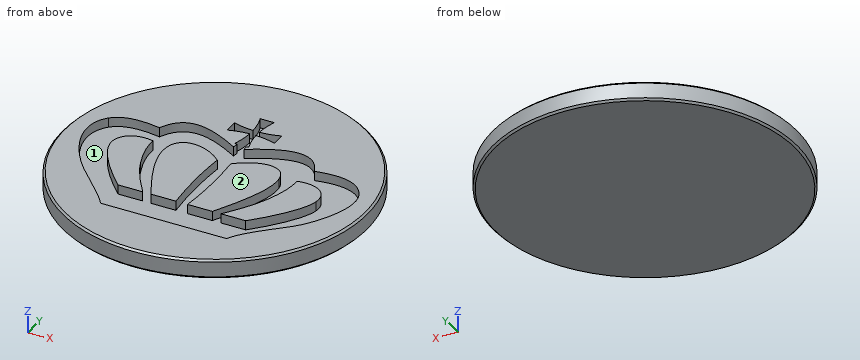
from build123d import *

# Parameters (mm, degrees)
POCKET_DEPTH = 1.25


with BuildPart() as part:
    # Sketch (on DatumPlane) → Revolution (revolve)
    with BuildSketch(Plane.YZ):
        Polygon((0, 0), (0, -2.5), (19.75, -2.5), (20, -2.25), (20, -0.25), (19.75, 0), align=None)
    revolve(axis=Axis((0, 0, 0), (0, 0, 1)))

    # Sketch005 → Pocket (cut)
    with BuildSketch(Plane.XY):
        with BuildLine():
            add(Edge.make_bspline(
                [(17.199673, 3.39502), (15.904895, 5.827494), (13.139208, 6.003619), (10.22119, 5.380033)],
                knots=[0, 0, 0, 0, 1, 1, 1, 1], degree=3))
            add(Edge.make_bspline(
                [(10.22119, 5.380033), (8.593193, 9.516663), (4.81358, 8.293289), (0.719788, 5.827494)],
                knots=[0, 0, 0, 0, 1, 1, 1, 1], degree=3))
            add(Edge.make_bspline(
                [(0.719788, 5.827494), (0.649422, 6.478351)],
                knots=[0, 0, 41.237809, 41.237809], degree=1))
            add(Edge.make_bspline(
                [(0.649422, 6.478351), (0.817118, 6.478351), (0.936272, 6.478351), (0.959337, 6.478351)],
                knots=[0, 0, 0, 0, 1, 1, 1, 1], degree=3))
            add(Edge.make_bspline(
                [(0.959337, 6.478351), (0.65764, 7.35953), (0.487238, 8.273468), (0.447992, 9.191671)],
                knots=[0, 0, 0, 0, 1, 1, 1, 1], degree=3))
            add(Edge.make_bspline(
                [(0.447992, 9.191671), (1.366194, 9.152423), (2.280132, 8.982021), (3.16131, 8.680326)],
                knots=[0, 0, 0, 0, 1, 1, 1, 1], degree=3))
            add(Edge.make_bspline(
                [(3.16131, 8.680326), (3.16131, 9.295984), (3.16131, 9.911639), (3.16131, 10.527295)],
                knots=[0, 0, 0, 0, 1, 1, 1, 1], degree=3))
            add(Edge.make_bspline(
                [(3.16131, 10.527295), (2.280132, 10.225599), (1.366194, 10.055198), (0.447992, 10.01595)],
                knots=[0, 0, 0, 0, 1, 1, 1, 1], degree=3))
            add(Edge.make_bspline(
                [(0.447992, 10.01595), (0.487238, 10.934154), (0.65764, 11.848094), (0.959337, 12.729271)],
                knots=[0, 0, 0, 0, 1, 1, 1, 1], degree=3))
            add(Edge.make_bspline(
                [(0.959337, 12.729271), (0.343681, 12.729271), (-0.271977, 12.729271), (-0.887634, 12.729271)],
                knots=[0, 0, 0, 0, 1, 1, 1, 1], degree=3))
            add(Edge.make_bspline(
                [(-0.887634, 12.729271), (-0.585937, 11.848092), (-0.415537, 10.934152), (-0.376289, 10.01595)],
                knots=[0, 0, 0, 0, 1, 1, 1, 1], degree=3))
            add(Edge.make_bspline(
                [(-0.376289, 10.01595), (-1.294491, 10.055198), (-2.20843, 10.2256), (-3.089607, 10.527295)],
                knots=[0, 0, 0, 0, 1, 1, 1, 1], degree=3))
            add(Edge.make_bspline(
                [(-3.089607, 10.527295), (-3.089607, 9.911639), (-3.089607, 9.295983), (-3.089607, 8.680326)],
                knots=[0, 0, 0, 0, 1, 1, 1, 1], degree=3))
            add(Edge.make_bspline(
                [(-3.089607, 8.680326), (-2.20843, 8.982023), (-1.294491, 9.152423), (-0.376289, 9.191671)],
                knots=[0, 0, 0, 0, 1, 1, 1, 1], degree=3))
            add(Edge.make_bspline(
                [(-0.376289, 9.191671), (-0.415537, 8.273468), (-0.585937, 7.359528), (-0.887634, 6.478351)],
                knots=[0, 0, 0, 0, 1, 1, 1, 1], degree=3))
            add(Edge.make_bspline(
                [(-0.887634, 6.478351), (-0.857358, 6.478351), (-0.732021, 6.478351), (-0.559748, 6.478351)],
                knots=[0, 0, 0, 0, 1, 1, 1, 1], degree=3))
            add(Edge.make_bspline(
                [(-0.559748, 6.478351), (-0.641636, 5.73229)],
                knots=[0, 0, 47.278241, 47.278241], degree=1))
            add(Edge.make_bspline(
                [(-0.641636, 5.73229), (-4.754593, 8.196928), (-8.497006, 9.617448), (-10.238244, 5.399072)],
                knots=[0, 0, 0, 0, 1, 1, 1, 1], degree=3))
            add(Edge.make_bspline(
                [(-10.238244, 5.399072), (-12.781371, 5.921869), (-15.207916, 5.846532), (-16.502695, 4.485108)],
                knots=[0, 0, 0, 0, 1, 1, 1, 1], degree=3))
            add(Edge.make_bspline(
                [(-16.502695, 4.485108), (-19.031136, 1.826532), (-16.97872, -3.140769), (-13.656084, -6.796618)],
                knots=[0, 0, 0, 0, 1, 1, 1, 1], degree=3))
            add(Edge.make_bspline(
                [(-13.656084, -6.796618), (-11.875374, -8.755908), (-9.359237, -11.018558), (-8.286551, -12.670729)],
                knots=[0, 0, 0, 0, 1, 1, 1, 1], degree=3))
            add(Edge.make_bspline(
                [(-8.286551, -12.670729), (8.364704, -12.670729)],
                knots=[0, 0, 1048.89791, 1048.89791], degree=1))
            add(Edge.make_bspline(
                [(8.364704, -12.670729), (9.202504, -10.757117), (12.053892, -8.352741), (13.859035, -6.607594)],
                knots=[0, 0, 0, 0, 1, 1, 1, 1], degree=3))
            add(Edge.make_bspline(
                [(13.859035, -6.607594), (15.505033, -5.01629), (18.826551, 0.33865), (17.199673, 3.39502)],
                knots=[0, 0, 0, 0, 1, 1, 1, 1], degree=3))
        make_face()
        with BuildLine():
            add(Edge.make_bspline(
                [(9.506608, 2.472112), (9.566387, 0.610416), (9.023596, -1.104203), (8.43058, -2.600588)],
                knots=[0, 0, 0, 0, 1, 1, 1, 1], degree=3))
            add(Edge.make_bspline(
                [(8.43058, -2.600588), (7.541741, -4.843446), (6.124803, -6.733903), (5.159797, -8.108826)],
                knots=[0, 0, 0, 0, 1, 1, 1, 1], degree=3))
            add(Edge.make_bspline(
                [(5.159797, -8.108826), (8.43058, -8.108826)],
                knots=[0, 0, 206.0336, 206.0336], degree=1))
            add(Edge.make_bspline(
                [(8.43058, -8.108826), (10.431762, -6.10195), (13.237427, -2.736096), (13.605757, -0.542472)],
                knots=[0, 0, 0, 0, 1, 1, 1, 1], degree=3))
            add(Edge.make_bspline(
                [(13.605757, -0.542472), (13.983087, 1.704704), (12.0088, 3.069906), (9.506608, 2.472112)],
                knots=[0, 0, 0, 0, 1, 1, 1, 1], degree=3))
        make_face(mode=Mode.SUBTRACT)
        with BuildLine():
            add(Edge.make_bspline(
                [(7.395219, 2.010956), (6.894209, 5.051162), (3.230589, 4.436291), (0.870734, 2.238688)],
                knots=[0, 0, 0, 0, 1, 1, 1, 1], degree=3))
            add(Edge.make_bspline(
                [(0.870734, 2.238688), (1.159981, -1.194989), (1.12982, -4.644717), (0.756864, -8.111676)],
                knots=[0, 0, 0, 0, 1, 1, 1, 1], degree=3))
            add(Edge.make_bspline(
                [(0.756864, -8.111676), (0.756864, -8.111677)],
                knots=[0, 0, 0.0001, 0.0001], degree=1))
            add(Edge.make_bspline(
                [(0.756864, -8.111677), (4.03619, -8.111677)],
                knots=[0, 0, 206.5717, 206.5717], degree=1))
            add(Edge.make_bspline(
                [(4.03619, -8.111677), (6.407437, -3.693701), (7.774117, -0.288253), (7.395219, 2.010956)],
                knots=[0, 0, 0, 0, 1, 1, 1, 1], degree=3))
        make_face(mode=Mode.SUBTRACT)
        with BuildLine():
            add(Edge.make_bspline(
                [(-9.516603, 2.472114), (-12.018792, 3.069908), (-13.99308, 1.704704), (-13.615756, -0.542474)],
                knots=[0, 0, 0, 0, 1, 1, 1, 1], degree=3))
            add(Edge.make_bspline(
                [(-13.615756, -0.542474), (-13.247425, -2.736097), (-10.441758, -6.101951), (-8.440576, -8.108828)],
                knots=[0, 0, 0, 0, 1, 1, 1, 1], degree=3))
            add(Edge.make_bspline(
                [(-8.440576, -8.108828), (-5.169793, -8.108828)],
                knots=[0, 0, 206.0336, 206.0336], degree=1))
            add(Edge.make_bspline(
                [(-5.169793, -8.108828), (-6.134802, -6.733903), (-7.551735, -4.843448), (-8.440576, -2.600593)],
                knots=[0, 0, 0, 0, 1, 1, 1, 1], degree=3))
            add(Edge.make_bspline(
                [(-8.440576, -2.600593), (-9.03359, -1.104203), (-9.576383, 0.610415), (-9.516603, 2.472114)],
                knots=[0, 0, 0, 0, 1, 1, 1, 1], degree=3))
        make_face(mode=Mode.SUBTRACT)
        with BuildLine():
            add(Edge.make_bspline(
                [(-0.905534, 2.238688), (-3.265394, 4.436293), (-6.929014, 5.051165), (-7.430021, 2.010958)],
                knots=[0, 0, 0, 0, 1, 1, 1, 1], degree=3))
            add(Edge.make_bspline(
                [(-7.430021, 2.010958), (-7.808915, -0.288249), (-6.442239, -3.693696), (-4.070992, -8.111676)],
                knots=[0, 0, 0, 0, 1, 1, 1, 1], degree=3))
            add(Edge.make_bspline(
                [(-4.070992, -8.111676), (-0.791666, -8.111676)],
                knots=[0, 0, 206.57171, 206.57171], degree=1))
            add(Edge.make_bspline(
                [(-0.791666, -8.111676), (-1.164621, -4.644717), (-1.194783, -1.194989), (-0.905534, 2.238688)],
                knots=[0, 0, 0, 0, 1, 1, 1, 1], degree=3))
        make_face(mode=Mode.SUBTRACT)
    extrude(amount=-POCKET_DEPTH, mode=Mode.SUBTRACT)


solid = part.part
Work out the finished part from the listing and answer in its coordinate system (mm). Face numbers are marked on the shaded views. Coordinates: 2 decimals unless noted, no trailing zeros. Write each question's results on one line, items separated by ' | '. Start each with the question number.
1) Flat-ended cylindrical pins translate along their axes: P1, Ø1, axis at x = 5.5, y = 1, coming from the +Z side; P2, Ø1.5, axis at x = -3.5, z = -1, coming from the -Y side. Find the tip coordinate at first contact, or state that the pin passes through.
2) The mould has two halves that part along X. Classify the marked faces 1 and 2: pulls with the +X half, pulls with the -X half, needs draft (parallel to the pull), parting line crosses it, or undercut.
3) Consider line 1 along X through (y, z) = (-7, -0.5) (1 decimal); line 2 along X through (y, z) = (1, -0.75); line 3 along Y through (x, z) = (1.5, -1.1). Determine where each line is inside the solid, lowest interval first.
Response values:
1) P1: stops at z = 0 | P2: stops at y = -19.81
2) face 1: undercut | face 2: needs draft
3) line 1: x = -18.7 to -13.5, -9.5 to -6, -4.7 to -0.9, 0.9 to 4.6, 5.9 to 9.5, 13.4 to 18.7 | line 2: x = -19.97 to -17.62, -13.47 to -9.44, -7.49 to -1, 0.96 to 7.45, 9.43 to 13.46, 17.62 to 19.97 | line 3: y = -19.94 to -12.67, -8.11 to 2.76, 6.28 to 9.09, 10.12 to 19.94
